Part print with two shaded views. Sizes in mm from the minimum x, y, z corner. A direction names the side the tool comes from. Coordinates: 2 decimals unless noted, no trailing zeros. Loops run counter-clockwise (first coordinate to the right, second up) from the corner with the lowest first, then second, coordinate; pieces in that order, holes last. Notation, with made-up numbers: (46, -1) -> (85, -1) arc R20 ccw to (85, 10) -> close; hole circle Ø7 at (-25.75, 16.5). An arc over 180 degrees is marked (long way). Return JSON: item names as keys, results as strings. Group by question number.
(1) Saw through at A-A on z = 5. Write the cut outline in (x, y), then the cut area to 3 significant figures.
(2) Tool access for the marked faces 1, 2 and 3: list every direction of +Z, -Z, +X, -X, +Y, -Y with a clear straight run to the whole face (end or side of a thin tool).
(3) Saw through at C-C on z = 26. Write the cut outline in (x, y), then the cut area to 4 significant figures.
(4) Probe L1, parallel to X at y = 1.1, z = 5; L2, parallel to X at y = 17.25, z = 30; L3, parallel to Z at x = 6, y = 1.15. List the from-to ranges inside material, lowest first.
(5) Saw through at B-B on x = 6. Write the cut outline in (y, z).
(6) Flat gauge pins, fed straight in: pin 1 Ø0.6 at (y, z) = (26.5, 27) entering from +X; pin 2 Ø2 at (x, z) = (26, 5) entering from -Y; pin 3 Ø2 at (y, z) = (17, 24) entering from -X; pin 4 Ø8 at (x, y) = (13.5, 20.5) entering from -Z. Where does each tip first touch, or does it go through?
(7) Saw through at D-D on x = 21. Write the cut outline in (y, z), then the cut area to 4 significant figures.
(8) Mould opens along Y. For the marked faces 4, 5, 6 and 7 say: pulls with the +Y half, pulls with the -Y half, needs draft (parallel to the pull), parting line crosses it, or undercut.
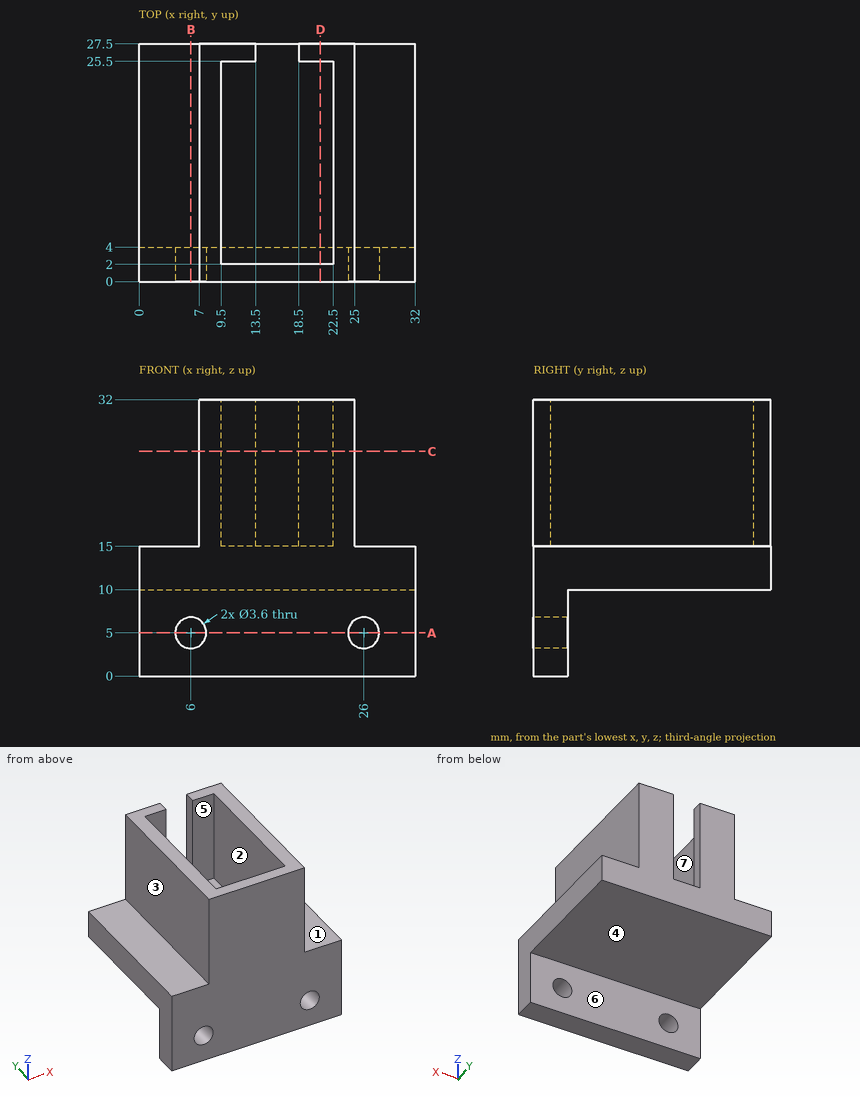
Geometry results:
{
 "1": {"outline": "(0, 0) -> (4.2, 0) -> (4.2, 4) -> (0, 4) -> close; (7.8, 0) -> (24.2, 0) -> (24.2, 4) -> (7.8, 4) -> close; (27.8, 0) -> (32, 0) -> (32, 4) -> (27.8, 4) -> close", "area": "99.2 mm²"},
 "2": {"face 1": "+Z, +X, +Y, -Y", "face 2": "+Z", "face 3": "+Z, -X, +Y, -Y"},
 "3": {"outline": "(7, 0) -> (25, 0) -> (25, 27.5) -> (18.5, 27.5) -> (18.5, 25.5) -> (22.5, 25.5) -> (22.5, 2) -> (9.5, 2) -> (9.5, 25.5) -> (13.5, 25.5) -> (13.5, 27.5) -> (7, 27.5) -> close", "area": "179.5 mm²"},
 "4": {"L1": "0 to 4.2, 7.8 to 24.2, 27.8 to 32", "L2": "7 to 9.5, 22.5 to 25", "L3": "0 to 3.2, 6.8 to 15"},
 "5": {"outline": "(0, 0) -> (4, 0) -> (4, 3.2) -> (0, 3.2) -> close; (0, 6.8) -> (4, 6.8) -> (4, 10) -> (27.5, 10) -> (27.5, 15) -> (0, 15) -> close"},
 "6": {"pin 1": "x = 25", "pin 2": "through", "pin 3": "x = 7", "pin 4": "z = 10"},
 "7": {"outline": "(0, 0) -> (4, 0) -> (4, 10) -> (27.5, 10) -> (27.5, 32) -> (25.5, 32) -> (25.5, 15) -> (2, 15) -> (2, 32) -> (0, 32) -> close", "area": "245.5 mm²"},
 "8": {"face 4": "needs draft", "face 5": "undercut", "face 6": "pulls with the +Y half", "face 7": "undercut"}
}
